Build history of the part. All positions in model axes, mm. Face numbers are marked on the shaded views. Coordinates: 2 decimals unless noted, no trailing zeros. Loops run counter-clockwise (first coordinate to the right, second up) from the corner with the lowest first, then second, coordinate; pieces in that order, holes last.
(1) Two-plate mould, pull along Y, no slides. Class the marked faces 1, 2 and 3: pulls with the +Y half, pulls with the -Y half, needs draft (parallel to the pull), parting line crosses it, or undercut.
(2) Slice it at A-A (y = 0). Give the number of separate pieces and of enclosed holes in the cut face, and give its area (3 significant figures).
(3) Wall check: L1, parallel to X at y = 0, z = 4.4; L2, parallel to Y at x = -4.5, z = 2.6. Give the ranges that are in metal, low to high.
(4) Slice it at B-B (z = 5). Give the cut face in (x, y).
(5) Flat gauge pins, fed straight in: P1, Ø2, axis at x = 3.5, z = 3, coming from the +Y side; P2, Ø2, axis at y = 5.5, z = 4.5, coming from the +X side; P3, Ø1.5, axis at y = -2.5, z = 2.5, coming from the -X side. Where does each tip first touch, or does it go through?
Autodesk Inventor part; units mm, degrees
ref_plane "YZ Plane" through (0, 0, 0) normal (1, 0, 0) x (0, 1, 0)
ref_plane "XZ Plane" through (0, 0, 0) normal (0, 1, 0) x (-1, 0, 0)
ref_plane "XY Plane" through (0, 0, 0) normal (0, 0, 1) x (1, 0, 0)
sketch "Sketch1" plane through (0, 0, 0) normal (0, 0, 1) x (1, 0, 0)
  circle A0 centre (0, 0) radius 3.25
  circle A1 centre (0, 0) radius 8
  dimension "d0" = 6.5
  dimension "d1" = 16
extrude "Extrusion1" add sketch "Sketch1" along normal blind 6
sketch "Sketch2" plane through (0, 0, 0) normal (1, 0, 0) x (0, 1, 0)
  circle A0 centre (0, 2.5) radius 1.25
  point P0 (0, 0)
  dimension "d4" = 2.5
extrude "Extrusion2" cut sketch "Sketch2" against normal blind 20
fillet "Fillet1" radius 0.5 1 edges at (-8, 0, 6)
fillet "Fillet2" radius 0.5 4 edges at (-7.9017, -1.25, 2.4978) (-8, 0, 0) (-3.25, 0, 0) (-3.25, 0, 6)
properties part number "6mmRingBracket"
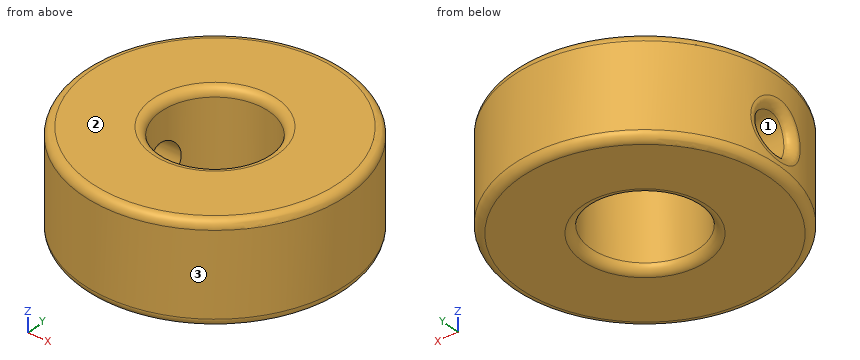
Response values:
1. face 1: undercut
1. face 2: needs draft
1. face 3: parting line crosses it
2. separate pieces: 3
2. enclosed holes: 0
2. area: 44.6 mm2
3. L1: x = -8 to -3.25, 3.25 to 8
3. L2: y = -6.61 to -1.25, 1.25 to 6.61
4. outline: circle Ø16 at (0, 0); hole circle Ø6.5 at (0, 0)
5. P1: stops at y = 7.6
5. P2: stops at x = 6.61
5. P3: stops at x = -7.79
